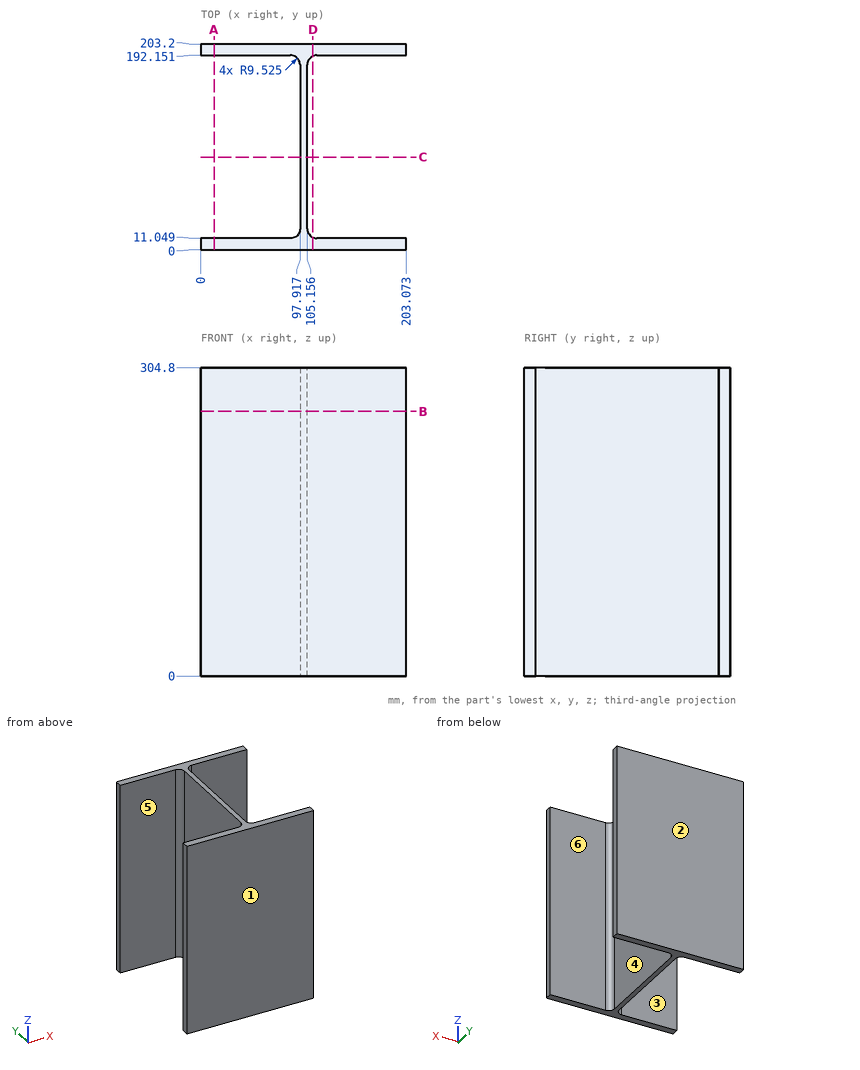
Answer from the drawing. Dimensions are ordinates in mm from the lowest x, y and z of the part. A direction names the side the tool comes from. Coordinates: 2 decimals unless noted, no trailing zeros. Order: outer loops, then holes, each group sorted by start corner. A loop starts at its lowest first (then second) coordinate and runs counter-clockwise, first axis right, second up. Notation, with made-up numbers: M -0.5,84.5 L 5.5,84.5 A30 cw 5.5,123.5 Z; hole C -9,72.5 d10. An arc over 180 degrees is marked long. Put each result on its own line as item: value. Start each with the question number.
Item 1: For the marked faces 5 and 6, determine the directions among +Z, -Z, +X, -X, +Y, -Y from which every point of the face is accessible in a straight line to the end or side of a thin tool.
Item 2: Section D-D, the plane x = 110.5 is taken. Determine the outline of the cut face in (y, z), plus the area to 3 significant figures.
Item 3: Given pin 1 Ø8 at (y, z) = (55.5, 243.5) entering from +X; pin 2 Ø1 at (y, z) = (54.5, 81.5) entering from -X; pin 3 Ø5 at (y, z) = (21.5, 219.5) entering from +X, each flat-ended and moving along its own axis, determine where each tip first touches the part or whether it passes through.
Item 4: Consider probe 1 along Y at (x, z) = (28.5, 201.5); probe 2 along Y at (x, z) = (113.5, 60.5); probe 3 along X at (y, z) = (30, 50.5). Determine where each line is inside the solid, lowest interval first. Write a range as [from, to].
Item 5: Section C-C, the plane y = 91.5 is taken. Determine the outline of the cut face in (x, z), plus the area to 3 significant figures.
Item 6: Section B-B, the plane z = 261.5 is taken. Determine the outline of the cut face in (x, y) (3 decimals), plus the area to 3 significant figures.
Item 7: Section A-A, the plane x = 13 is taken. Determine the outline of the cut face in (y, z).
Item 8: The mould has two halves that part along Y. Classify the marked faces 1, 2, 3 and 4: +Y half, -Y half, draft (parallel to the pull), parting line (faces both ways), or undercut.
Computed:
1. face 5: +Z, -Z, -X
1. face 6: +Z, -Z, +X
2. outline: M 0,0 L 12.02,0 L 12.02,304.8 L 0,304.8 Z; M 191.18,0 L 203.2,0 L 203.2,304.8 L 191.18,304.8 Z
2. area: 7,320 mm2
3. pin 1: stops at x = 105.16
3. pin 2: stops at x = 97.92
3. pin 3: stops at x = 105.29
4. probe 1: y = [0, 11.05], [192.15, 203.2]
4. probe 2: y = [0, 11.12], [192.08, 203.2]
4. probe 3: x = [97.92, 105.16]
5. outline: M 97.92,0 L 105.16,0 L 105.16,304.8 L 97.92,304.8 Z
5. area: 2,210 mm2
6. outline: M 0,0 L 203.073,0 L 203.073,11.049 L 114.681,11.049 A9.525 cw 105.156,20.574 L 105.156,182.626 A9.525 cw 114.681,192.151 L 203.073,192.151 L 203.073,203.2 L 0,203.2 L 0,192.151 L 88.392,192.151 A9.525 cw 97.917,182.626 L 97.917,20.574 A9.525 cw 88.392,11.049 L 0,11.049 Z
6. area: 5,880 mm2
7. outline: M 0,0 L 11.05,0 L 11.05,304.8 L 0,304.8 Z; M 192.15,0 L 203.2,0 L 203.2,304.8 L 192.15,304.8 Z
8. face 1: -Y half
8. face 2: +Y half
8. face 3: undercut
8. face 4: undercut
